Read the model definition and answer for the solid it produces. Units are mm, in the model's axes. Coordinates: 2 decimals unless noted, no trailing zeros. Order: outer loops, then holes, each group sorted by start corner. A loop starts at its lowest first (then second) coordinate and runs counter-clockwise, first axis right, second up. Notation, with made-up numbers: M -13,12.25 L 25,12.25 A31 ccw 25,39.25 Z; hole C 67.25,88 d10. An arc over 180 degrees is marked long. Put each result on its own line as item: value.
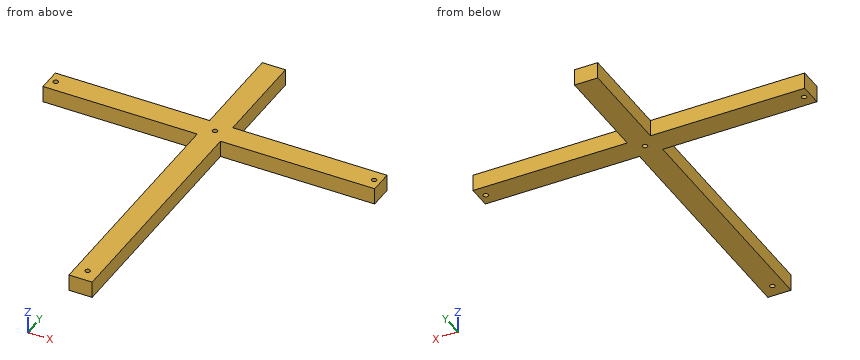
from build123d import *

# Parameters (mm, degrees)
F0_R     = 0.1905
F1_DEPTH = 1.27


with BuildPart() as f1:
    # F0 (on Top) → F1 (new body)
    with BuildSketch(Plane.XY):
        Polygon((-0.889, 0.889), (-12.7, 0.889), (-12.7, -0.889), (-0.889, -0.889), (-0.889, -19.431), (0.889, -19.431), (0.889, -0.889), (12.7, -0.889), (12.7, 0.889), (0.889, 0.889), (0.889, 8.509), (-0.889, 8.509), align=None)
        with Locations((0, -18.415)):
            Circle(F0_R, mode=Mode.SUBTRACT)
        with Locations((-12.192, 0)):
            Circle(F0_R, mode=Mode.SUBTRACT)
        Circle(F0_R, mode=Mode.SUBTRACT)
        with Locations((12.192, 0)):
            Circle(F0_R, mode=Mode.SUBTRACT)
    extrude(amount=F1_DEPTH)


solid = f1.part
Q1. Find section B-B on y = -6.25. Write down the section's boundary in (x, z).
Answers below:
outline: M -0.89,0 L 0.89,0 L 0.89,1.27 L -0.89,1.27 Z
Q2. Consider line 1 along Y through (x, z) = (0, 0.45); line 2 along X through (y, z) = (-12.25, 0.8). Determine where each line is inside the solid, lowest interval first.
Answers below:
line 1: y = -19.43 to -18.61, -18.22 to -0.19, 0.19 to 8.51
line 2: x = -0.89 to 0.89
Q3. Given pin 1 (0.6 mm diameter, centred on x = 5, z = 0.5, fed in from -Y); pin 2 (0.6 mm diameter, centred on y = -9, z = 0.5, fed in from -X); pin 3 (0.6 mm diameter, centred on x = -5, z = 1, fed in from +Y); pin 4 (2 mm diameter, centred on x = -3.5, y = -5, fed in from +Z), each flat-ended and moving along its own axis, determine where each tip first touches the part or whether it passes through.
Answers below:
pin 1: stops at y = -0.89
pin 2: stops at x = -0.89
pin 3: stops at y = 0.89
pin 4: passes through
Q4. Find section A-A on z = 0.25. Write down the section's boundary in (x, y) (1 decimal).
Answers below:
outline: M -12.7,-0.9 L -0.9,-0.9 L -0.9,-19.4 L 0.9,-19.4 L 0.9,-0.9 L 12.7,-0.9 L 12.7,0.9 L 0.9,0.9 L 0.9,8.5 L -0.9,8.5 L -0.9,0.9 L -12.7,0.9 Z; hole C -12.2,0 d0.4; hole C 0,-18.4 d0.4; hole C 0,0 d0.4; hole C 12.2,0 d0.4
